Verification items for this drawing (mm, ordinates from the low corner). A direction names the side the tool comes from. Round coordinates to 2 decimals unless told otherwise and drop trailing zeros. Order: outer loops, then holes, each group sorted by start corner. A loop starts at its lowest first (then second) coordinate and runs counter-clockwise, first axis right, second up. Notation, with made-up numbers: (-38.75, 23) -> (-33.75, 23) arc R35 cw to (-33.75, 59) -> close; hole circle Ø9 at (-19, 54). An arc over 180 degrees is marked (long way). Answer in a Markdown table with one row per item. Add a question column.
1. Depth check by flat-ended pin: P1, Ø5, axis at x = 48, z = 53.5, coming from the +Y side; P2, Ø6.5, axis at x = 27.5, z = 27.5, coming from the +Y side. Enter the tip coordinate at first touch or a pass-through.
2. Material ranges on L1, parallel to X at y = 36, z = 55.5; L2, parallel to Z at x = 53.5, y = 53.5; L3, parallel to Z at x = 89.5, y = 13.5, recorded low to high. Write a range as from..to.
3. Sectioned sample at D-D, the plane y = 92.5. Record the boundary of the cut face in (x, z).
4. Draft check along X on the marked faces 1, 2 and 3. Enter one of: +X half, -X half, draft (parallel to the pull), parting line (faces both ways), or undercut.
5. Sectioned sample at A-A, the plane y = 34. Record the boundary of the cut face in (x, z), then the cut area to 4 significant figures.
6. Sectioned sample at B-B, the plane z = 77.5. Count the separate pieces of the cut face and the enclosed holes in it, then the cut area to 3 significant figures.
7. Access from +Z, -Z, +X, -X, +Y, -Y to the whole of each face (thin tool, end or side, straight path). Record for the marked faces 4 and 5.
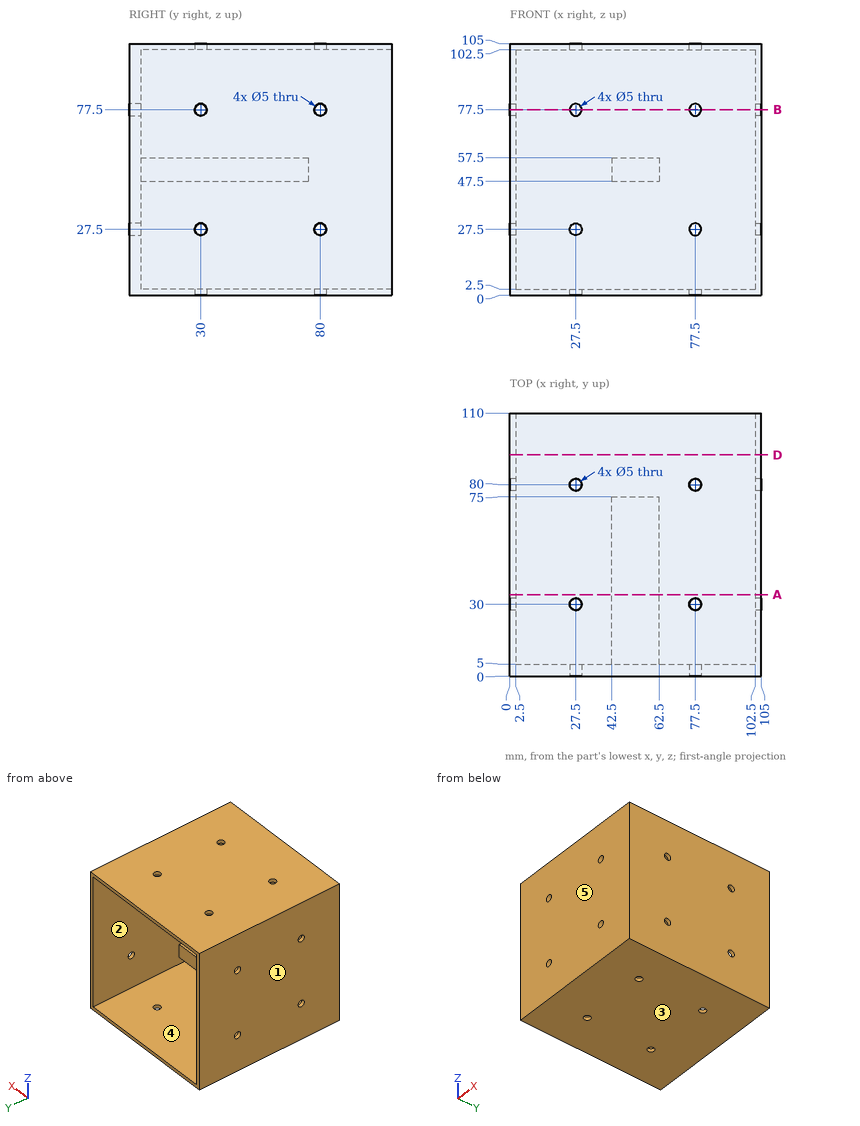
Answer key:
| question | item | result |
|---|---|---|
| 1 | P1 | stops at y = 75 |
| 1 | P2 | stops at y = 5 |
| 2 | L1 | x = 0..2.5, 42.5..62.5, 102.5..105 |
| 2 | L2 | z = 0..2.5, 47.5..57.5, 102.5..105 |
| 2 | L3 | z = 0..2.5, 102.5..105 |
| 3 | outline | (0, 0) -> (105, 0) -> (105, 105) -> (0, 105) -> close; hole (2.5, 2.5) -> (102.5, 2.5) -> (102.5, 102.5) -> (2.5, 102.5) -> close |
| 4 | face 1 | -X half |
| 4 | face 2 | undercut |
| 4 | face 3 | draft |
| 5 | outline | (0, 0) -> (105, 0) -> (105, 105) -> (0, 105) -> close; (42.5, 47.5) -> (62.5, 47.5) -> (62.5, 57.5) -> (42.5, 57.5) -> close; hole (2.5, 2.5) -> (102.5, 2.5) -> (102.5, 102.5) -> (2.5, 102.5) -> close |
| 5 | area | 1,225 mm² |
| 6 | separate pieces | 7 |
| 6 | enclosed holes | 0 |
| 6 | area | 950 mm² |
| 7 | face 4 | +Y |
| 7 | face 5 | +Z, -Z, +X, -X, -Y |
